Verification items for the finished model (mm, model axes). A direction names the side the tool comes from. Coordinates: 2 decimals unless noted, no trailing zeros. Order: outer loops, then holes, each group sorted by start corner. A loop starts at its lowest first (then second) coordinate and runs counter-clockwise, first axis right, second up. Notation, with made-up numbers: M -26.75,50 L -7.75,50 A25 ccw -7.75,89 Z; hole C 73,76.25 d10. An arc over 180 degrees is marked long. Return JSON: item names as keys, results as strings. Group by question number.
1. Material ranges on line 1 along Y through (x, z) = (1.75, -0.75); line 2 along Y through (x, z) = (1.75, 2.25); line 3 along X through (y, z) = (10.25, 0.25), recorded low to high.
2. Mould release check, pull along Y, two halves, no side actions. Record for faces 1 (the flat face through (0, 22.689, 1)), 2 (the cylindrical face through (-0.079, 2.796, 1.798)), 3 (the flat face through (-2, 3.289, 0)), 4 (the cylindrical face through (-2.024, 5.216, -1.291)): +Y half, -Y half, draft (parallel to the pull), parting line (faces both ways), or undercut.
3. Section check B-B, the plane y = 19.75. Record the cut outline in (x, z).
4. Set-up check for faces 5 (the cylindrical face through (-0.26, -0.09, 1.17)), 6 (the flat face through (0, 2.289, -3)), 7 (the cylindrical face through (-4.2, 0.5, 0)), 8 (the cylindrical face through (-0.079, 14.694, 1.798)): record each of +Z, -Z, +X, -X, +Y, -Y from which the full face is reachable in a straight line by a thin tool's end or side.
5. Gauge pin test, flat ends, axial feed: pin 1 (1.5 mm diameter, centred on x = 2.5, z = -1.5, fed in from +Y); pin 2 (1.5 mm diameter, centred on y = 16, z = 1.5, fed in from -X); pin 3 (1.6 mm diameter, centred on x = 0, z = 0, fed in from -Y). Record the tip position at first contact, or that the pin passes through.
```python
from build123d import *

# Parameters (mm, degrees)
SKETCH2_R                 = 0.5
CUT_EXTRUDE2_DEPTH        = 21.603397778
F_2_0MM_DOWEL_HOLE1_D     = 2
F_2_0MM_DOWEL_HOLE1_DEPTH = 2
F_2_0MM_DOWEL_HOLE1_TIP   = 0.600860619
CUT_EXTRUDE3_DEPTH        = 21.603397778
CUT_EXTRUDE4_DEPTH        = 5
CUT_EXTRUDE4_DEPTH_BACK   = 18
SCALE1_SCALE              = 1.2


with BuildPart() as part:
    # Sketch1 → Revolve2 (revolve)
    with BuildSketch(Plane.XY, mode=Mode.PRIVATE) as revolve2_sk:
        with BuildLine():
            Line((0, 0), (-3.5, 0))
            Line((-3.5, 0), (-3.5, 3))
            Line((-3.5, 3), (-1.5, 3))
            Line((-1.5, 3), (-1.5, 3.833209081))
            Line((-1.5, 3.833209081), (-2, 3.833209081))
            Line((-2, 3.833209081), (-2, 7))
            Line((-2, 7), (-1.5, 7))
            Line((-1.5, 7), (-1.5, 19.5))
            ThreePointArc((-1.5, 19.5), (-1.353553391, 19.853553391), (-1, 20))
            Line((-1, 20), (0, 20))
            Line((0, 20), (0, 0))
        make_face()
    revolve(revolve2_sk.sketch.rotate(Axis((0, 7, 0), (0, 1, 0)), 270), axis=Axis((0, 7, 0), (0, 1, 0)))

    # Sketch2 → Cut-Extrude2 (cut, through all)
    with BuildSketch(Plane(origin=(0, 20, 0), x_dir=(1, 0, 0), z_dir=(0, 1, 0))):
        with Locations(Location((0, 0, 0), (0, 0, 270))):
            Circle(SKETCH2_R)
    extrude(amount=-CUT_EXTRUDE2_DEPTH, mode=Mode.SUBTRACT)

    # Ø2.0mm Dowel Hole1
    with Locations(Plane(origin=(0, 0, 0), x_dir=(-1, 0, 0), z_dir=(0, -1, 0))):
        with Locations((0, 0)):
            Hole(F_2_0MM_DOWEL_HOLE1_D / 2, depth=F_2_0MM_DOWEL_HOLE1_DEPTH)
            with Locations((0, 0, -(F_2_0MM_DOWEL_HOLE1_DEPTH + F_2_0MM_DOWEL_HOLE1_TIP / 2))):  # 118° drill point
                Cone(0, F_2_0MM_DOWEL_HOLE1_D / 2, F_2_0MM_DOWEL_HOLE1_TIP, mode=Mode.SUBTRACT)

    # Sketch6 → Cut-Extrude3 (cut, through all)
    with BuildSketch(Plane(origin=(0, 20, 0), x_dir=(1, 0, 0), z_dir=(0, 1, 0))):
        with BuildLine():
            Line((1.802775638, -3), (-1.802775638, -3))
            ThreePointArc((-1.802775638, -3), (0, -3.5), (1.802775638, -3))
        make_face()
        with BuildLine():
            Line((-1.861759264, 2.963756475), (1.802775638, 3))
            ThreePointArc((1.802775638, 3), (-0.034614525, 3.499828829), (-1.861759264, 2.963756475))
        make_face()
    extrude(amount=-CUT_EXTRUDE3_DEPTH, mode=Mode.SUBTRACT)

    # Sketch7 → Cut-Extrude4 (cut, two sides: drawn at the far end of the back side and taken through both)
    with BuildSketch(Plane.XY.offset(-CUT_EXTRUDE4_DEPTH_BACK)):
        with BuildLine():
            Line((-4.156062939, 2.838931077), (-4.156062939, 3.239498592))
            Line((-4.156062939, 3.239498592), (-1.5, 3.239498592))
            Line((-1.5, 3.239498592), (-1.5, 2.979046191))
            ThreePointArc((-1.5, 2.979046191), (-2.828899089, 2.925435476), (-4.156062939, 2.838931077))
        make_face()
        with BuildLine():
            Line((4.156062939, 3.239498592), (1.5, 3.239498592))
            Line((1.5, 3.239498592), (1.5, 2.979046191))
            ThreePointArc((1.5, 2.979046191), (2.828899089, 2.925435476), (4.156062939, 2.838931077))
            Line((4.156062939, 2.838931077), (4.156062939, 3.239498592))
        make_face()
    extrude(amount=CUT_EXTRUDE4_DEPTH + CUT_EXTRUDE4_DEPTH_BACK, mode=Mode.SUBTRACT)


with BuildPart() as part_1:
    # Scale1: scaled about (0.000542722, 6.55250098, 0.00261842)
    add(part.part.scale(SCALE1_SCALE).moved(Location((-0.000108544, -1.310500196, -0.000523684))))


solid = part_1.part
```
Answers follow:
{
 "1": {"line 1": "-1.31 to 2.29, 3.29 to 7.09", "line 2": "-1.31 to 2.29", "line 3": "-1.78 to -0.55, 0.55 to 1.78"},
 "2": {"face 1": "+Y half", "face 2": "undercut", "face 3": "undercut", "face 4": "draft"},
 "3": {"outline": "C 0,0 d3.6; hole C 0,0 d1.2"},
 "4": {"face 5": "-Y", "face 6": "-Z", "face 7": "-X, +Y, -Y", "face 8": "+Y"},
 "5": {"pin 1": "y = 7.09", "pin 2": "x = -1.64", "pin 3": "y = 1.33"}
}
